Read the model definition and answer for the solid it produces. Units are mm, in the model's axes. A direction names the side the tool comes from. Coordinates: 2 decimals unless noted, no trailing zeros. Answer as a JSON object with one key per item and string values. Group by question number.
Q1. Each of these flat-tipped pins is pushed along its axis until it touches: P1, Ø0.5, axis at x = -4, y = 104, coming from the +Z side; P2, Ø0.9, axis at y = -104, z = 4, coming from the +X side; P3, Ø4.5, axis at x = 0, z = -5.5, coming from the -Y side. Where does it stop, or does it pass through?
Q2. Determine the mould class of faces 4 (the flat face through (-7.5, 1, 5)), 5 (the cylindrical face through (3.5, 1.44, -0.06)), 6 (the flat face through (0, -107.5, 0)) for opening direction X: released by +X, released by -X, zero draft, split by the parting line, or undercut.
Q3. For faces 1 (the cylindrical face through (-3.502, 1.442, 0.099)), 2 (the cylindrical face through (-3, -104, 0)), 3 (the cylindrical face through (0, 104, 3)), determine the directions among +Z, -Z, +X, -X, +Y, -Y from which every point of the face is accessible in a straight line to the end or side of a thin tool.
Q4. Straight lines are drawn through the part: line 1 along X through (y, z) = (4.5, 5.5); line 2 along Z through (x, y) = (5.5, 104.5); line 3 along Z through (x, y) = (-6.5, 98.5). For each, find the intervals that lie inside material, in ascending order. Write a range as [from, to].
from build123d import *

# Parameters (mm, degrees)
EXTRUDE_1_DEPTH     = 103
EXTRUDE_2_DEPTH     = 2
EXTRUDE_3_DEPTH     = 2
CUT_EXTRUDE_1_DEPTH = 2.5
FILLET_1_R          = 0.1
FILLET_2_R          = 0.2
FILLET_3_R          = 0.2


with BuildPart() as part:
    # 草图1 → 凸台-拉伸1 (new body)
    with BuildSketch(Plane(origin=(0, 0, 0), x_dir=(1, 0, 0), z_dir=(0, 1, 0))):
        with BuildLine():
            Line((-7.5, 7.5), (-1.5, 7.5))
            Line((-1.5, 7.5), (-1.5, 6.822875656))
            ThreePointArc((-1.5, 6.822875656), (0, 3.5), (1.5, 6.822875656))
            Line((1.5, 6.822875656), (1.5, 7.5))
            Line((1.5, 7.5), (7.5, 7.5))
            Line((7.5, 7.5), (7.5, 1.5))
            Line((7.5, 1.5), (6.822875656, 1.5))
            ThreePointArc((6.822875656, 1.5), (3.5, 0), (6.822875656, -1.5))
            Line((6.822875656, -1.5), (7.5, -1.5))
            Line((7.5, -1.5), (7.5, -7.5))
            Line((7.5, -7.5), (1.5, -7.5))
            Line((1.5, -7.5), (1.5, -6.822875656))
            ThreePointArc((1.5, -6.822875656), (0, -3.5), (-1.5, -6.822875656))
            Line((-1.5, -6.822875656), (-1.5, -7.5))
            Line((-1.5, -7.5), (-7.5, -7.5))
            Line((-7.5, -7.5), (-7.5, -1.5))
            Line((-7.5, -1.5), (-6.822875656, -1.5))
            ThreePointArc((-6.822875656, -1.5), (-3.5, 0), (-6.822875656, 1.5))
            Line((-6.822875656, 1.5), (-7.5, 1.5))
            Line((-7.5, 1.5), (-7.5, 7.5))
        make_face()
    extrude_1 = extrude(amount=EXTRUDE_1_DEPTH)

    # 草图2 → 凸台-拉伸2 (add)
    with BuildSketch(Plane(origin=(0, 103, 0), x_dir=(1, 0, 0), z_dir=(0, 1, 0))):
        with BuildLine():
            Line((-7, 7), (-7, 2))
            ThreePointArc((-7, 2), (-3, 0), (-7, -2))
            Line((-7, -2), (-7, -7))
            Line((-7, -7), (-2, -7))
            ThreePointArc((-2, -7), (0, -3), (2, -7))
            Line((2, -7), (7, -7))
            Line((7, -7), (7, -2))
            ThreePointArc((7, -2), (3, 0), (7, 2))
            Line((7, 2), (7, 7))
            Line((7, 7), (2, 7))
            ThreePointArc((2, 7), (0, 3), (-2, 7))
            Line((-2, 7), (-7, 7))
        make_face()
    extrude_2 = extrude(amount=EXTRUDE_2_DEPTH)

    # 草图3 → 凸台-拉伸3 (add, symmetric)
    with BuildSketch(Plane(origin=(0, 0, 0), x_dir=(0, 0, -1), z_dir=(1, 0, 0))):
        with BuildLine():
            Line((-1.5, 105), (1.5, 105))
            Line((1.5, 105), (1.5, 105.677124344))
            ThreePointArc((1.5, 105.677124344), (1.780042303, 106.088161527), (1.95, 106.555590279))
            Line((1.95, 106.555590279), (1.95, 107.5))
            Line((1.95, 107.5), (-1.95, 107.5))
            Line((-1.95, 107.5), (-1.95, 106.555590279))
            ThreePointArc((-1.95, 106.555590279), (-1.780042303, 106.088161527), (-1.5, 105.677124344))
            Line((-1.5, 105.677124344), (-1.5, 105))
        make_face()
    extrude_3 = extrude(amount=EXTRUDE_3_DEPTH, both=True)

    # 草图4 → 切除-拉伸1 (cut, symmetric)
    with BuildSketch(Plane.XY):
        with BuildLine():
            Line((1.5, 105), (1.5, 105.677124344))
            ThreePointArc((1.5, 105.677124344), (1.780042303, 106.088161527), (1.95, 106.555590279))
            Line((1.95, 106.555590279), (1.95, 107.5))
            Line((1.95, 107.5), (2.5, 107.5))
            Line((2.5, 107.5), (2.5, 105))
            Line((2.5, 105), (1.5, 105))
        make_face()
        with BuildLine():
            Line((-1.5, 105), (-1.5, 105.677124344))
            ThreePointArc((-1.5, 105.677124344), (-1.780042303, 106.088161527), (-1.95, 106.555590279))
            Line((-1.95, 106.555590279), (-1.95, 107.5))
            Line((-1.95, 107.5), (-2.5, 107.5))
            Line((-2.5, 107.5), (-2.5, 105))
            Line((-2.5, 105), (-1.5, 105))
        make_face()
    cut_extrude_1 = extrude(amount=CUT_EXTRUDE_1_DEPTH, both=True, mode=Mode.SUBTRACT)

    # 镜向1: 凸台-拉伸1, 凸台-拉伸2, 凸台-拉伸3, 切除-拉伸1 across plane
    add(extrude_1.mirror(Plane.ZX))
    add(extrude_2.mirror(Plane.ZX))
    add(extrude_3.mirror(Plane.ZX))
    add(cut_extrude_1.mirror(Plane.ZX), mode=Mode.SUBTRACT)

    # 圆角1
    fillet_1_edges = [part.edges().sort_by_distance(p)[0] for p in [
        (0, 107.5, -1.95),
        (0, 107.5, 1.95),
        (-1.95, 107.5, 0),
        (1.95, 107.5, 0),
        (0, -107.5, 1.95),
        (0, -107.5, -1.95),
        (-1.95, -107.5, 0),
        (1.95, -107.5, 0),
    ]]
    fillet(fillet_1_edges, radius=FILLET_1_R)

    # 圆角2
    fillet_2_edges = [part.edges().sort_by_distance(p)[0] for p in [
        (-4.5, -105, -7),
        (-7, -104, -7),
        (-2, -104, -7),
        (4.5, -105, -7),
        (2, -104, -7),
        (7, -105, -4.5),
        (7, -104, -7),
        (7, -104, -2),
        (7, -105, 4.5),
        (7, -104, 2),
        (4.5, -105, 7),
        (7, -104, 7),
        (2, -104, 7),
        (-4.5, -105, 7),
        (-2, -104, 7),
        (-7, -105, 4.5),
        (-7, -104, 7),
        (-7, -104, 2),
        (-7, -105, -4.5),
        (-7, -104, -2),
        (-2, 104, -7),
        (-7, 104, -7),
        (-7, 104, -2),
        (-7, 104, 2),
        (-7, 104, 7),
        (-2, 104, 7),
        (2, 104, 7),
        (7, 104, 7),
        (7, 104, 2),
        (7, 104, -2),
        (7, 104, -7),
        (2, 104, -7),
        (-4.5, 105, -7),
        (-7, 105, -4.5),
        (-7, 105, 4.5),
        (-4.5, 105, 7),
        (4.5, 105, 7),
        (7, 105, 4.5),
        (7, 105, -4.5),
        (4.5, 105, -7),
    ]]
    fillet(fillet_2_edges, radius=FILLET_2_R)

    # 圆角3
    fillet_3_edges = [part.edges().sort_by_distance(p)[0] for p in [
        (-7.5, 0, -7.5),
        (-1.5, 0, -7.5),
        (1.5, 0, -7.5),
        (7.5, 0, -7.5),
        (7.5, 0, -1.5),
        (7.5, 0, 1.5),
        (7.5, 0, 7.5),
        (1.5, 0, 7.5),
        (-1.5, 0, 7.5),
        (-7.5, 0, 7.5),
        (-7.5, 0, 1.5),
        (-6.822875656, 0, -1.5),
        (-7.5, 0, -1.5),
    ]]
    fillet(fillet_3_edges, radius=FILLET_3_R)


solid = part.part
Final values:
{
 "1": {"P1": "stops at z = 7", "P2": "stops at x = 7", "P3": "stops at y = -103"},
 "2": {"face 4": "released by -X", "face 5": "undercut", "face 6": "zero draft"},
 "3": {"face 1": "+Y, -Y", "face 2": "-Y", "face 3": "+Y"},
 "4": {"line 1": "x = [-7.5, -2], [2, 7.5]", "line 2": "z = [-7, -2.5], [2.5, 7]", "line 3": "z = [-7.5, -1.73], [1.73, 7.5]"}
}
